```python
from build123d import *
from build123d.topology import SkipClean

# Parameters (mm, degrees)
SKETCH1_R           = 3.81
SKETCH1_R_2         = 1.4605
SKETCH1_R_3         = 2.159
BOSS_EXTRUDE1_DEPTH = 2.286
BOSS_EXTRUDE2_START = 3.556
SKETCH3_W           = 8.798430976
SKETCH3_H           = 8.128
SKETCH3_R           = 2.159
BOSS_EXTRUDE2_DEPTH = 3.556
FILLET1_R           = 3.81
FILLET2_R           = 3.81
FILLET3_R           = 0.635


with BuildPart() as part:
    # Sketch1 → Boss-Extrude1 (new body)
    with BuildSketch(Plane(origin=(0, 0, 0), x_dir=(1, 0, 0), z_dir=(0, 1, 0))):
        with BuildLine():
            Line((-12.328815677, 3.048), (-21.980815677, 3.048))
            Line((-21.980815677, 3.048), (-21.980815677, -5.08))
            Line((-21.980815677, -5.08), (-11.639742265, -5.08))
            ThreePointArc((-11.639742265, -5.08), (12.654605425, 1.072828757), (-12.328815677, 3.048))
        make_face()
        with Locations(Location((0, 0, 0), (0, 0, 270))):
            Circle(SKETCH1_R, mode=Mode.SUBTRACT)
        with Locations(Location((9.525, 0, 0), (0, 0, 270))):
            Circle(SKETCH1_R_2, mode=Mode.SUBTRACT)
        with Locations(Location((-9.525, 0, 0), (0, 0, 270))):
            Circle(SKETCH1_R_2, mode=Mode.SUBTRACT)
        with Locations(Location((-17.78, -1.016, 0), (0, 0, 270))):
            Circle(SKETCH1_R_3, mode=Mode.SUBTRACT)
    extrude(amount=BOSS_EXTRUDE1_DEPTH)

    # Sketch3 → Boss-Extrude2 (add)
    with SkipClean():  # the faces are left unmerged after this step: merging them gives an invalid solid
        with BuildSketch(Plane.XZ.offset(BOSS_EXTRUDE2_START)):
            with Locations((-17.581600189, 1.016)):
                Rectangle(SKETCH3_W, SKETCH3_H)
            with Locations(Location((-17.78, 1.016, 0), (0, 0, 270))):
                Circle(SKETCH3_R, mode=Mode.SUBTRACT)
        extrude(amount=-BOSS_EXTRUDE2_DEPTH)

    # Fillet1
    fillet1_edges = [part.edges().sort_by_distance(p)[0] for p in [
        (-21.980815677, -1.778, 5.08),
        (-21.980815677, -1.778, -3.048),
    ]]
    fillet(fillet1_edges, radius=FILLET1_R)

    # Fillet2
    # the kernel refuses this fillet: 3.81 mm, written as the material it adds along each edge
    with BuildSketch(Plane(origin=(-12.328815677, -6.723594375, -3.048), x_dir=(-1, 0, 0), z_dir=(0, 1, 0))) as fillet2_piece_1_section:
        with BuildLine():
            CenterArc((2.68943775, -3.81), FILLET2_R, 90, 65.456460121)
            ThreePointArc((-0.776313041, -2.227384615), (-0.336332546, -1.13175458), (0, 0))
            Line((0, 0), (2.68943775, 0))
        make_face()
    fillet2_piece_1 = extrude(amount=9.009594375, mode=Mode.PRIVATE)
    fillet2_piece_1 = split(fillet2_piece_1, bisect_by=Plane(origin=(-13.789984069, 0, -3.128673841), z_dir=(0, -1, 0)), keep=Keep.TOP, mode=Mode.PRIVATE)
    fillet2_piece_1 = split(fillet2_piece_1, bisect_by=Plane(origin=(-13.789984069, -3.556, -3.128673841), z_dir=(0, 1, 0)), keep=Keep.TOP, mode=Mode.PRIVATE)
    fillet2_piece_1 = split(fillet2_piece_1, bisect_by=Plane(origin=(-13.182384701, -1.778, -3.128673841), z_dir=(-1, 0, 0)), keep=Keep.TOP, mode=Mode.PRIVATE)
    add(fillet2_piece_1)
    with BuildSketch(Plane(origin=(-12.328815677, 0, -3.048), x_dir=(-1, 0, 0), z_dir=(0, 1, 0))) as fillet2_piece_2_section:
        with BuildLine():
            CenterArc((2.68943775, -3.81), FILLET2_R, 90, 65.456460121)
            ThreePointArc((-0.776313041, -2.227384615), (-0.336332546, -1.13175458), (0, 0))
            Line((0, 0), (2.68943775, 0))
        make_face()
    fillet2_piece_2 = extrude(amount=2.286, mode=Mode.PRIVATE)
    fillet2_piece_2 = split(fillet2_piece_2, bisect_by=Plane(origin=(-13.182384701, 1.143, -3.128673841), z_dir=(-1, 0, 0)), keep=Keep.TOP, mode=Mode.PRIVATE)
    add(fillet2_piece_2)
    with BuildSketch(Plane(origin=(-12.328815677, 0, -3.048), x_dir=(-1, 0, 0), z_dir=(0, 1, 0))) as fillet2_piece_3_section:
        with BuildLine():
            CenterArc((2.68943775, -3.81), FILLET2_R, 90, 65.456460121)
            ThreePointArc((-0.776313041, -2.227384615), (-0.336332546, -1.13175458), (0, 0))
            Line((0, 0), (2.68943775, 0))
        make_face()
    fillet2_piece_3 = extrude(amount=2.286, mode=Mode.PRIVATE)
    fillet2_piece_3 = split(fillet2_piece_3, bisect_by=Plane(origin=(-13.182384701, 1.143, -3.680280143), z_dir=(1, 0, 0)), keep=Keep.TOP, mode=Mode.PRIVATE)
    add(fillet2_piece_3)
    with BuildSketch(Plane(origin=(-11.639742265, -5.681026739, 5.08), x_dir=(0.47068197991323696, 0, 0.8823029376495101), z_dir=(0, 1, 0))) as fillet2_piece_4_section:
        with BuildLine():
            CenterArc((2.291991427, -3.798252976), FILLET2_R, 94.500395957, 57.421029607)
            Line((-1.069582765, -2.004954632), (0, 0))
            ThreePointArc((0, 0), (0.996518012, -0.039156748), (1.993036024, 0))
        make_face()
    fillet2_piece_4 = extrude(amount=7.967026739, mode=Mode.PRIVATE)
    fillet2_piece_4 = split(fillet2_piece_4, bisect_by=Plane(origin=(-13.504288869, 0, 5.055827312), z_dir=(0, -1, 0)), keep=Keep.TOP, mode=Mode.PRIVATE)
    fillet2_piece_4 = split(fillet2_piece_4, bisect_by=Plane(origin=(-13.504288869, -3.556, 5.055827312), z_dir=(0, 1, 0)), keep=Keep.TOP, mode=Mode.PRIVATE)
    fillet2_piece_4 = split(fillet2_piece_4, bisect_by=Plane(origin=(-13.182384701, -1.778, 5.055827312), z_dir=(-1, 0, 0)), keep=Keep.TOP, mode=Mode.PRIVATE)
    add(fillet2_piece_4)
    with BuildSketch(Plane(origin=(-11.639742265, 0, 5.08), x_dir=(0.47068197991323696, 0, 0.8823029376495101), z_dir=(0, 1, 0))) as fillet2_piece_5_section:
        with BuildLine():
            CenterArc((2.291991427, -3.798252976), FILLET2_R, 94.500395957, 57.421029607)
            Line((-1.069582765, -2.004954632), (0, 0))
            ThreePointArc((0, 0), (0.996518012, -0.039156748), (1.993036024, 0))
        make_face()
    fillet2_piece_5 = extrude(amount=2.286, mode=Mode.PRIVATE)
    fillet2_piece_5 = split(fillet2_piece_5, bisect_by=Plane(origin=(-13.182384701, 1.143, 5.488267474), z_dir=(1, 0, 0)), keep=Keep.TOP, mode=Mode.PRIVATE)
    add(fillet2_piece_5)
    with BuildSketch(Plane(origin=(-11.639742265, 0, 5.08), x_dir=(0.47068197991323696, 0, 0.8823029376495101), z_dir=(0, 1, 0))) as fillet2_piece_6_section:
        with BuildLine():
            CenterArc((2.291991427, -3.798252976), FILLET2_R, 94.500395957, 57.421029607)
            Line((-1.069582765, -2.004954632), (0, 0))
            ThreePointArc((0, 0), (0.996518012, -0.039156748), (1.993036024, 0))
        make_face()
    fillet2_piece_6 = extrude(amount=2.286, mode=Mode.PRIVATE)
    fillet2_piece_6 = split(fillet2_piece_6, bisect_by=Plane(origin=(-13.182384701, 1.143, 5.055827312), z_dir=(-1, 0, 0)), keep=Keep.TOP, mode=Mode.PRIVATE)
    add(fillet2_piece_6)

    # Fillet3
    fillet3_edges = [part.edges().sort_by_distance(p)[0] for p in [
        (-13.182384701, -3.556, 0.815529295),
        (-13.182384701, 0, 0.815529295),
    ]]
    fillet(fillet3_edges, radius=FILLET3_R)


solid = part.part
```
Could you check a few things on this model? Use its own coordinates, in mm. A direction names the side the tool comes from. Coordinates: 2 decimals unless noted, no trailing zeros. Order: outer loops, then holes, each group sorted by start corner. A loop starts at its lowest first (then second) coordinate and runs counter-clockwise, first axis right, second up. Notation, with made-up numbers: M 60,50.5 L 90,50.5 A22 cw 90,75.5 Z; hole C 9.5,22 d6. An arc over 180 degrees is marked long. Use one line per item in the form item = value. Start each with the question number.
1. Suppose I cut it at C-C on x = 0. Write out the boundary of the cut face in (y, z).
2. On a 3-axis mill with a long thin cutter (end or side, diameter ignored), from which of +Z, -Z, +X, -X, +Y, -Y can I reach the whole of each face in a straight line? I mean faces 1 (the flat face through (-13.182, -2, 1)), 2 (the cylindrical face through (-20.894, -0.594, 3.934)). Say none if no direction works.
3. For pin 1 (1.5 mm diameter, centred on x = -14, y = 0, fed in from +Z); pin 2 (3 mm diameter, centred on y = -2.5, z = 3, fed in from -X); pin 3 (1 mm diameter, centred on x = 3, z = -3, fed in from -Y), each with a flat end and sliding along its axis, tell me the tip position at first contact or that it passes through.
4. Please list where these lines run through material, in increasing order: line 1 (X direction, y = 1.9, z = 2.25); line 2 (X direction, y = 0.9, z = 2.5); line 3 (X direction, y = 0.95, z = 0) (1 decimal).
5. Suppose I cut it at B-B on z = -0.25. Write out the boundary of the cut face in (x, y) (3 decimals).
6. Suppose I cut it at D-D on z = 11.25. Write out the boundary of the cut face in (x, y), then the cut area to 3 significant figures.
7. We'd pull the mould along Z, two halves only. Please class faces 3 (the cylindrical face through (8.1, 1.13, -0.32)), 4 (the flat face through (-16, -1, 5.08)), 5 (the flat face through (-17, -1, -3.048)): +Z half, -Z half, draft (parallel to the pull), parting line (faces both ways), or undercut.
8. Suppose I cut it at A-A on x = -17.78. Write out the boundary of the cut face in (y, z) (3 decimals), then the cut area to 3 significant figures.
Geometry says:
q1.outline = M 0,-12.7 L 2.29,-12.7 L 2.29,-3.81 L 0,-3.81 Z; M 0,3.81 L 2.29,3.81 L 2.29,12.7 L 0,12.7 Z
q2.face_1 = +Z, -Z, +X, -Y
q2.face_2 = +Z, -X, +Y, -Y
q3.pin_1 = 5.14
q3.pin_2 = -21.97
q3.pin_3 = 0
q4.line_1 = -21.85 to -19.55, -16.01 to -3.07, 3.07 to 12.5
q4.line_2 = -21.78 to -19.35, -16.21 to -2.88, 2.88 to 12.45
q4.line_3 = -21.9 to -19.7, -15.9 to -11, -8.1 to -3.8, 3.8 to 8.1, 11 to 12.7
q5.outline = M -21.844,-3.556 L -19.529,-3.556 L -19.529,2.286 L -21.844,2.286 Z; M -16.031,-3.556 L -13.817,-3.556 A0.635 ccw -13.182,-2.921 L -13.182,-0.635 A0.635 cw -12.547,0 L -10.964,0 L -10.964,2.286 L -16.031,2.286 Z; M -8.086,0 L -3.802,0 L -3.802,2.286 L -8.086,2.286 Z; M 3.802,0 L 8.086,0 L 8.086,2.286 L 3.802,2.286 Z; M 10.964,0 L 12.698,0 L 12.698,2.286 L 10.964,2.286 Z
q6.outline = M -5.89,0 L 5.89,0 L 5.89,2.29 L -5.89,2.29 Z
q6.area = 26.9 mm^2
q7.face_3 = undercut
q7.face_4 = +Z half
q7.face_5 = -Z half
q8.outline = M -3.556,-3.048 L 2.286,-3.048 L 2.286,-1.143 L -3.556,-1.143 Z; M -3.556,3.175 L 2.286,3.175 L 2.286,5.08 L -3.556,5.08 Z
q8.area = 22.3 mm^2
